from build123d import *

# Parameters (mm, degrees)
POCKET_DEPTH = 2.56


with BuildPart() as part:
    # Sketch → Revolve (revolve)
    with BuildSketch(Plane.YZ):
        with BuildLine():
            Line((1.499, 0), (2.75, 0))
            Line((2.75, 0), (2.75, 2.97229))
            ThreePointArc((2.75, 2.97229), (2.741884, 2.991884), (2.72229, 3))
            Line((2.72229, 3), (0, 3))
            Line((0, -22), (0, 3))
            Line((1, -22), (0, -22))
            Line((1.5, -21.5), (1, -22))
            Line((1.5, -4), (1.5, -21.5))
            Line((1.499, 0), (1.5, -4))
        make_face()
    revolve(axis=Axis((0, 0, 0), (0, 0, 1)))

    # Sketch001 → Pocket (cut)
    with BuildSketch(Plane.XY.offset(3)):
        Polygon((1.478017, 0), (0.739008, 1.28), (-0.739008, 1.28), (-1.478017, 0), (-0.739008, -1.28), (0.739008, -1.28), align=None)
    extrude(amount=-POCKET_DEPTH, mode=Mode.SUBTRACT)


solid = part.part
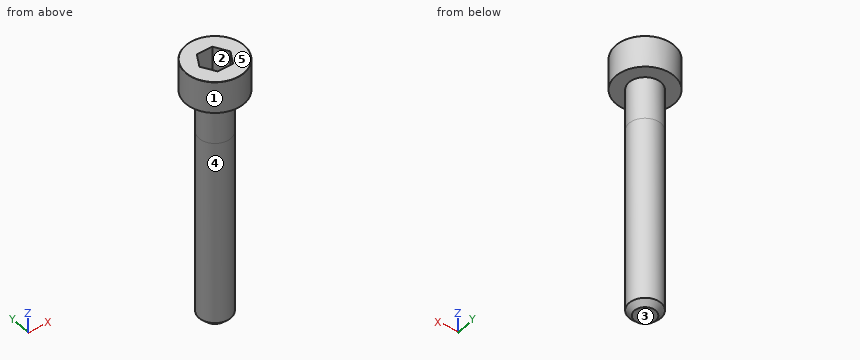
Verification items for the finished model (mm, model axes). Face numbers are marked on the shaded views. A direction names the side the tool comes from. Coordinates: 2 decimals unless noted, no trailing zeros. Order: outer loops, then holes, each group sorted by start corner. A loop starts at its lowest first (then second) coordinate and runs counter-clockwise, first axis right, second up. Notation, with made-up numbers: M -3,-11.5 L 43,-11.5 A28 ccw 43,7.5 Z; hole C 88.5,68.5 d7. An arc over 180 degrees is marked long. One line per item, written item: value. Start each with the question number.
Item 1: Access from +Z, -Z, +X, -X, +Y, -Y to the whole of each face (thin tool, end or side, straight path). Record for the marked faces 4 and 5.
Item 2: Sectioned sample at B-B on z = -4.75. Record the cut outline in (x, y).
Item 3: Sectioned sample at A-A on z = 0.75. Record the cut outline in (x, y).
Item 4: Thickness scan on probe 1 along Z at (x, y) = (-0.7, -0.45); probe 2 along Z at (x, y) = (-1.3, -1.2); probe 3 along X at (y, z) = (-0.2, -5.25). Record the ranges inside material, lowest first.
Item 5: Mould release check, pull along X, two halves, no side actions. Record for the marked faces 1, 2 and 3: pulls with the +X half, pulls with the -X half, needs draft (parallel to the pull), parting line crosses it, or undercut.
Item 6: Depth check by flat-ended pin: P1, Ø3, axis at x = -1, z = -14, coming from the -Y side; P2, Ø0.7, axis at x = 0.5, z = 1, coming from the -Y side; P3, Ø1, axis at y = -1, z = -13, coming from the +X side. Enter the tip coordinate at first touch or a pass-through.
Calculated:
1. face 4: -Z
1. face 5: +Z, +X, -X, +Y, -Y
2. outline: C 0,0 d3
3. outline: C 0,0 d5.5; hole M -1.48,0 L -0.74,-1.28 L 0.74,-1.28 L 1.48,0 L 0.74,1.28 L -0.74,1.28 Z
4. probe 1: -22 to 0.44
4. probe 2: 0 to 3
4. probe 3: -1.49 to 1.49
5. face 1: parting line crosses it
5. face 2: undercut
5. face 3: needs draft
6. P1: y = -1.5
6. P2: y = -2.75
6. P3: x = 1.41
